The model under review builds one solid part; all positions refer to its coordinate system, in mm. A direction names the side the tool comes from. Coordinates: 2 decimals unless noted, no trailing zeros. Loops run counter-clockwise (first coordinate to the right, second up) from the corner with the lowest first, then second, coordinate; pieces in that order, holes last. Notation, with made-up numbers: (60.25, 12.5) - (100.25, 12.5) arc R15 cw to (100.25, 29.5) - close; hole circle Ø1 at (54.25, -20.75). An arc over 180 degrees is marked (long way). Use a Markdown table: item, result. Add a question column.
1) For faces 1 (the flat face through (44.45, 0, -3)), 2 (the flat face through (-8.6, -16.4, 0)), 3 (the flat face through (1, -15.875, 8)), 4 (the flat face through (46, 0, -3.175)), list the 3-axis set-ups (+Z, -Z, +X, -X, +Y, -Y) from which the entire face can be reached by the end or side of a thin tool; tool diameter is ignored.
2) Add section A-A, the plane x = 14. Give the boundary of the cut face in (y, z) (3 decimals), and give its area (3 significant figures).
3) Add section B-B, the plane z = -17. Give the boundary of the cut face in (x, y) (3 decimals).
4) Clearance check with flat-ended pins moving along their axes: pin 1 (8 mm diameter, centred on x = 7.5, y = 14, fed in from -Z); pin 2 (11 mm diameter, centred on y = -4.5, z = -26.5, fed in from -X). State where each tip first meets the part, or that it passes through.
5) Add section C-C, the plane y = -6.5. Give the boundary of the cut face in (x, z) (3 decimals).
6) To check wall thickness, follow L1, parallel to X at y = -5, z = 7 (3 decimals); L2, parallel to Y at x = 6, z = 12 (3 decimals); L3, parallel to X at y = -16, z = -24 (3 decimals). State the ranges of each line that lie inside material, in increasing order. Write a range as [from, to].
7) The part is to be moulded in two halves that separate along X. For faces 5 (the flat face through (-1, 15.875, 8)), 6 (the flat face through (46, -15.24, -32)), 7 (the flat face through (-47.625, 0, 8)), 8 (the flat face through (-44.45, 0, 8)), say which applies: pulls with the +X half, pulls with the -X half, needs draft (parallel to the pull), parting line crosses it, or undercut.
```python
from build123d import *

# Parameters (mm, degrees)
F1_DEPTH = 15.875
F3_DEPTH = 3.175


with BuildPart() as f1:
    # F0 (on Top) → F1 (new body)
    with BuildSketch(Plane.XY):
        Polygon((-47.625, 18.49301), (-44.45, 15.875), (0, 15.875), (44.45, 15.875), (47.625, 18.49301), align=None)
        Polygon((-44.45, 0), (-44.45, 15.875), (-47.625, 18.49301), (-47.625, -18.49301), (-44.45, -15.875), align=None)
        Polygon((47.625, 18.49301), (44.45, 15.875), (44.45, 0), (44.45, -15.875), (47.625, -18.49301), align=None)
        Polygon((0, -15.875), (-44.45, -15.875), (-47.625, -18.49301), (47.625, -18.49301), (44.45, -15.875), align=None)
    extrude(amount=F1_DEPTH)

    # F2 (on face) → F3 (join)
    with BuildSketch(Plane.YZ.offset(47.625)):
        Polygon((18.49301, 0), (-18.49301, 0), (-15.24, -3.175), (15.24, -3.175), (15.24, -60.325), (18.49301, -63.5), align=None)
        Polygon((-15.24, -3.175), (-18.49301, 0), (-18.49301, -63.5), (-15.24, -60.325), align=None)
        Polygon((-15.24, -60.325), (-18.49301, -63.5), (18.49301, -63.5), (15.24, -60.325), align=None)
    extrude(amount=-F3_DEPTH)


solid = f1.part
```
From the geometry:
| question | item | result |
|---|---|---|
| 1 | face 1 | -Z |
| 1 | face 2 | -Z, -X, +Y, -Y |
| 1 | face 3 | +Z, -Z |
| 1 | face 4 | +X, -X |
| 2 | outline | (-18.493, 0) - (-15.875, 0) - (-15.875, 15.875) - (-18.493, 15.875) - close; (15.875, 0) - (18.493, 0) - (18.493, 15.875) - (15.875, 15.875) - close |
| 2 | area | 83.1 mm^2 |
| 3 | outline | (44.45, -18.493) - (47.625, -18.493) - (47.625, -15.24) - (44.45, -15.24) - close; (44.45, 15.24) - (47.625, 15.24) - (47.625, 18.493) - (44.45, 18.493) - close |
| 4 | pin 1 | stops at z = 0 |
| 4 | pin 2 | passes through |
| 5 | outline | (-47.625, 0) - (-44.45, 0) - (-44.45, 15.875) - (-47.625, 15.875) - close; (44.45, -63.5) - (47.625, -63.5) - (47.625, -60.325) - (44.45, -60.325) - close; (44.45, -3.175) - (47.625, -3.175) - (47.625, 15.875) - (44.45, 15.875) - close |
| 6 | L1 | x = [-47.625, -44.45], [44.45, 47.625] |
| 6 | L2 | y = [-18.493, -15.875], [15.875, 18.493] |
| 6 | L3 | x = [44.45, 47.625] |
| 7 | face 5 | undercut |
| 7 | face 6 | needs draft |
| 7 | face 7 | pulls with the -X half |
| 7 | face 8 | undercut |
